Print and shaded views of the part. All mm, measured from the part's lowest x, y and z. A direction names the side the tool comes from. Coordinates: 2 decimals unless noted, no trailing zeros. Order: outer loops, then holes, each group sorted by start corner. A loop starts at its lowest first (then second) coordinate and runs counter-clockwise, first axis right, second up. Notation, with made-up numbers: (60.5, -19.75) -> (77.5, -19.75) arc R10 cw to (77.5, -5.75) -> close; hole circle Ø5 at (40, -1.75). An arc over 180 degrees is marked (long way). Write item = value, one per line. Start each with the question number.
Q1. Cut at D-D, the plane x = 72. List the corners of the cut face in (y, z).
Q2. Flat gauge pins, fed straight in: pin 1 (3 mm diameter, centred on y = 26, z = 43.5, fed in from -X); pin 2 (3 mm diameter, centred on y = 30.5, z = 24, fed in from +X); pin 3 (4 mm diameter, centred on y = 45.5, z = 34.5, fed in from +X). Where does each tip first touch, or does it go through?
Q3. Cut at B-B, the plane x = 49. List the corners of the cut face in (y, z).
Q4. Wall check: line 1 (Y direction, x = 53.5, z = 10); line 2 (Z direction, x = 11, y = 57.5); line 3 (Y direction, x = 62, z = 29) (1 decimal). Give the ranges that are in metal, low to high. Write a range as from..to.
Q5. Mould opens along Y. For the marked faces 5, 6 and 7 say: +Y half, -Y half, draft (parallel to the pull), parting line (faces both ways), or undercut.
Q6. Cut at A-A, the plane z = 32.5. List the corners of the cut face in (x, y).
Q7. 3-axis set-ups, long thin cutter, end or side, ignore diameter. For the marked faces 1, 2, 3 and 4: which of +Z, -Z, +X, -X, +Y, -Y reach the whole face in a straight line?
Q8. Cut at C-C, the plane y = 68.5. List the corners of the cut face in (x, z), plus the area to 3 significant figures.
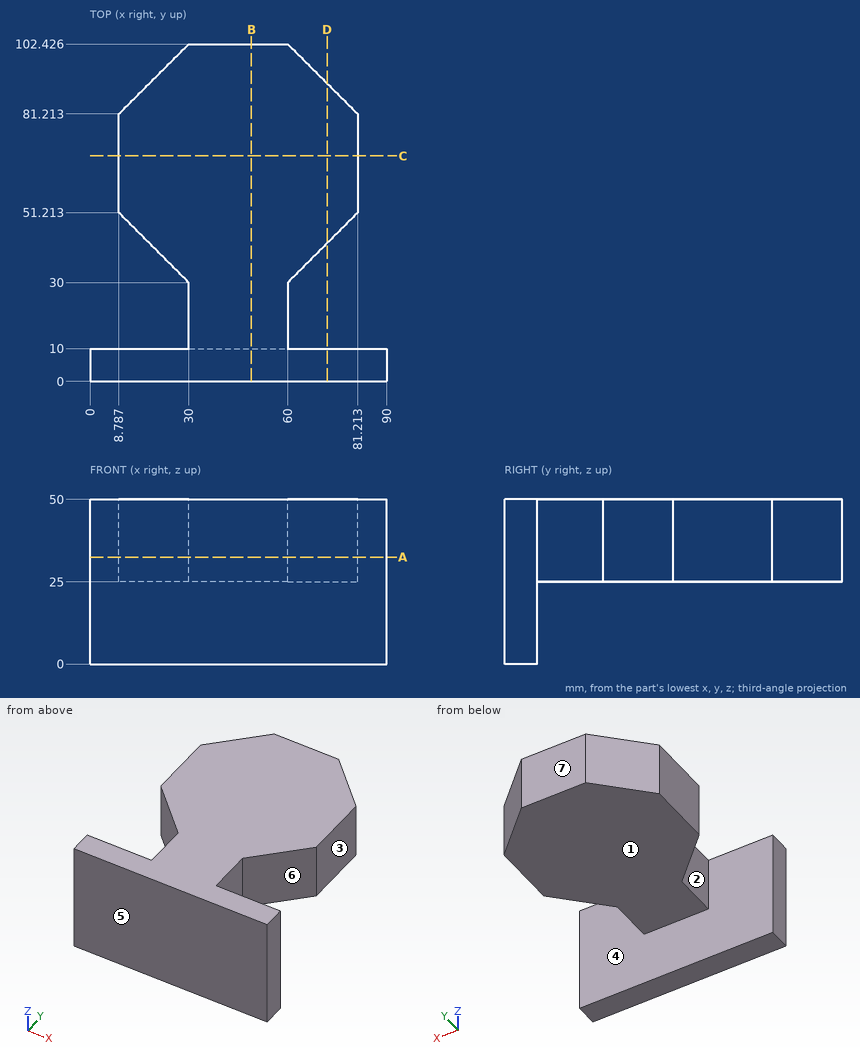
Here are the results:
q1.outline = (0, 0) -> (10, 0) -> (10, 50) -> (0, 50) -> close; (42, 25) -> (90.43, 25) -> (90.43, 50) -> (42, 50) -> close
q2.pin_1 = 30
q2.pin_2 = 61.62
q2.pin_3 = 77.5
q3.outline = (0, 0) -> (10, 0) -> (10, 25) -> (102.43, 25) -> (102.43, 50) -> (0, 50) -> close
q4.line_1 = 0..10
q4.line_2 = 25..50
q4.line_3 = 0..10, 32..100.4
q5.face_5 = -Y half
q5.face_6 = undercut
q5.face_7 = +Y half
q6.outline = (0, 0) -> (90, 0) -> (90, 10) -> (60, 10) -> (60, 30) -> (81.21, 51.21) -> (81.21, 81.21) -> (60, 102.43) -> (30, 102.43) -> (8.79, 81.21) -> (8.79, 51.21) -> (30, 30) -> (30, 10) -> (0, 10) -> close
q7.face_1 = -Z, +X, -X, +Y
q7.face_2 = +Z, -Z, -X
q7.face_3 = +Z, -Z, +X, +Y
q7.face_4 = -Z
q8.outline = (8.79, 25) -> (81.21, 25) -> (81.21, 50) -> (8.79, 50) -> close
q8.area = 1,810 mm²
